Part model, mm, in its own coordinate system. Face numbers are marked on the shaded views. Give positions to 0.01 mm unless a question says otherwise; leave off trailing zeros. Write each loop counter-clockwise with the first axis right and the second up, starting at its lowest first coordinate (ties: lowest second). Pieces come first, ordered by that corner, then holes. Notation, with made-up numbers: M 22,-16 L 45,-16 A30 cw 45,10 Z; hole C -20,40 d11. An arc over 180 degrees is marked long. Answer as CSV lines item,"result". Start each with the question number.
Item 1: Band-saw the part on A-A, the plane x = -769. List the corners of the cut face in (y, z).
Item 2: Two-plate mould, pull along Y, no slides. Class the marked faces 1, 2, 3 and 4: +Y half, -Y half, draft (parallel to the pull), parting line (faces both ways), or undercut.
Item 3: Band-saw the part on C-C, the plane y = -164.5. List the corners of the cut face in (x, z), then the cut area to 3 significant figures.
Item 4: Band-saw the part on D-D, the plane y = 4. List the corners of the cut face in (x, z).
Item 5: Wall check: L1, parallel to X at y = -350.5, z = -61; L2, parallel to Y at x = -415.5, z = -33; L3, parallel to Z at x = -567.5, y = 29. Give the ranges that are in metal, low to high. Write a range as from..to.
Item 6: Band-saw the part on B-B, the plane z = -19. List the corners of the cut face in (x, y).
Item 7: Pin check, flat tip, straight feed: pin 1 (1 mm diameter, centred on x = -261.5, y = -85.5, fed in from -Z). Stop position of the tip, or through.
from build123d import *

# Parameters (mm, degrees)
F0_W     = 1219.2
F0_H     = 609.6
F1_DEPTH = 12.7
F2_W     = 38.1
F2_H     = 533.4
F3_DEPTH = 88.9
F4_W     = 254
F4_H     = 101.6
F5_DEPTH = 0.254


# Not quite as in the source:
# - a length typed as a fraction of an inch, garbled in the dataset ("3 / 203.2 mm" for 3/8 in), is restored


with BuildPart() as f1:
    # F0 (on Top) → F1 (new body)
    with BuildSketch(Plane.XY):
        with Locations((-609.6, -177.4520107999)):
            Rectangle(F0_W, F0_H)
    extrude(amount=F1_DEPTH)

    # F2 (on face) → F3 (join)
    with BuildSketch(Plane(origin=(0, 0, 0), x_dir=(1, 0, 0), z_dir=(0, 0, -1))):
        Polygon((-1181.1, -89.2479892001), (-1219.2, -89.2479892001), (-1219.2, -127.3479892001), (0, -127.3479892001), (0, -89.2479892001), (-38.1, -89.2479892001), (-1167.365193367, -89.2479892001), align=None)
        Polygon((0, 482.2520107999), (-1219.2, 482.2520107999), (-1219.2, 444.1520107999), (-1181.1, 444.1520107999), (-1167.365193367, 444.1520107999), (-38.1, 444.1520107999), (0, 444.1520107999), align=None)
        with Locations((-1200.15, 177.4520107999)):
            Rectangle(F2_W, F2_H)
        with Locations((-19.05, 177.4520107999)):
            Rectangle(F2_W, F2_H)
    extrude(amount=F3_DEPTH)

    # F4 (on face) → F5 (join)
    with BuildSketch(Plane.XY.offset(12.7)):
        with Locations((-609.6, -177.4520107999)):
            Rectangle(F4_W, F4_H)
    extrude(amount=F5_DEPTH)


solid = f1.part
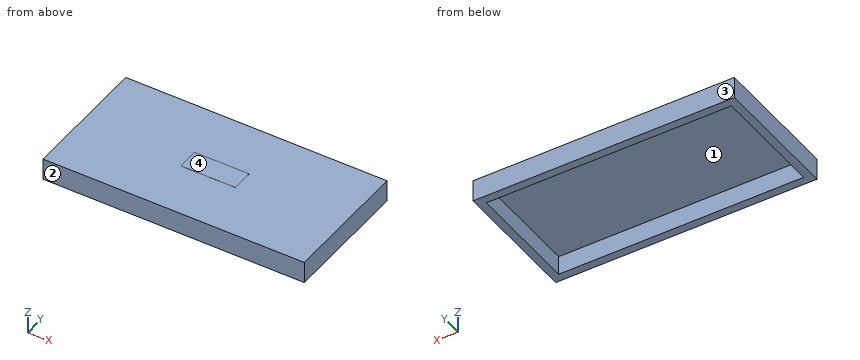
Output:
1,outline,"M -482.25,-88.9 L -444.15,-88.9 L -444.15,0 L 89.25,0 L 89.25,-88.9 L 127.35,-88.9 L 127.35,12.7 L -482.25,12.7 Z"
2,face 1,"undercut"
2,face 2,"-Y half"
2,face 3,"+Y half"
2,face 4,"draft"
3,outline,"M -1219.2,-88.9 L -1181.1,-88.9 L -1181.1,0 L -38.1,0 L -38.1,-88.9 L 0,-88.9 L 0,12.7 L -482.6,12.7 L -482.6,12.95 L -736.6,12.95 L -736.6,12.7 L -1219.2,12.7 Z"
3,area,"22,300 mm²"
4,outline,"M -1219.2,-88.9 L -1181.1,-88.9 L -1181.1,0 L -38.1,0 L -38.1,-88.9 L 0,-88.9 L 0,12.7 L -1219.2,12.7 Z"
5,L1,"-1219.2..-1181.1, -38.1..0"
5,L2,"-482.25..-444.15, 89.25..127.35"
5,L3,"0..12.7"
6,outline,"M -1219.2,-482.25 L 0,-482.25 L 0,127.35 L -1219.2,127.35 Z; hole M -1181.1,-444.15 L -38.1,-444.15 L -38.1,89.25 L -1181.1,89.25 Z"
7,pin 1,"z = 0"
